For this review, take the finished solid that the model builds, in its own axes (mm). A direction names the side the tool comes from. Round coordinates to 2 decimals unless told otherwise and drop trailing zeros. Write each loop counter-clockwise with the first axis right and the second up, starting at its lowest first coordinate (ties: lowest second). Pieces come first, ordered by that corner, then holes. Notation, with made-up numbers: M 37.25,19 L 69.25,19 A14 cw 69.25,24 Z; hole C 42.5,-8 d6. An arc over 180 degrees is marked long. Write each question's results on one line, items separated by ' | '. Start each with the question number.
```python
from build123d import *

# Parameters (mm, degrees)
SKETCH1_R                = 6
SKETCH1_R_2              = 4.5
BOSS_EXTRUDE1_DEPTH      = 2
SKETCH1_5_R              = 21
SKETCH1_5_R_2            = 6
BOSS_EXTRUDE3_DEPTH      = 2.75
SKETCH2_R                = 1.75
CUT_EXTRUDE1_DEPTH       = 4.5
CIRPATTERN1_COUNT        = 3
SKETCH9_W                = 60
SKETCH9_H                = 11
BOSS_EXTRUDE7_DEPTH      = 15
BOSS_EXTRUDE7_DEPTH_BACK = 2.75
CUT_EXTRUDE3_REACH       = 13
SKETCH10_R               = 2.5
FILLET4_R                = 3
FILLET5_R                = 5


with BuildPart() as part:
    # Sketch1 → Boss-Extrude1 (new body)
    with BuildSketch(Plane(origin=(0, 0, 0), x_dir=(1, 0, 0), z_dir=(0, 1, 0))):
        Circle(SKETCH1_R)
        Circle(SKETCH1_R_2, mode=Mode.SUBTRACT)
    extrude(amount=BOSS_EXTRUDE1_DEPTH)

    # Sketch1<5> → Boss-Extrude3 (add)
    with BuildSketch(Plane(origin=(0, 0, 0), x_dir=(1, 0, 0), z_dir=(0, 1, 0))):
        Circle(SKETCH1_5_R)
        Circle(SKETCH1_5_R_2, mode=Mode.SUBTRACT)
    extrude(amount=BOSS_EXTRUDE3_DEPTH)

    # Sketch2 → Cut-Extrude1 (cut)
    with BuildSketch(Plane(origin=(0, 2.75, 0), x_dir=(1, 0, 0), z_dir=(0, 1, 0))):
        with Locations((0, -13.5)):
            Circle(SKETCH2_R)
    cut_extrude1 = extrude(amount=-CUT_EXTRUDE1_DEPTH, mode=Mode.SUBTRACT)

    # CirPattern1: Cut-Extrude1 ×3 about axis
    cirpattern1_axis = Axis((0, 0, 0), (0, 1, 0))
    for i in range(1, CIRPATTERN1_COUNT):
        add(cut_extrude1.rotate(cirpattern1_axis, i * 360 / CIRPATTERN1_COUNT), mode=Mode.SUBTRACT)

    # Sketch9 → Boss-Extrude7 (add, two sides)
    with BuildSketch(Plane.XZ) as boss_extrude7_sk:
        with Locations((0, -19.5)):
            Rectangle(SKETCH9_W, SKETCH9_H)
    extrude(amount=BOSS_EXTRUDE7_DEPTH)
    extrude(boss_extrude7_sk.sketch, amount=-BOSS_EXTRUDE7_DEPTH_BACK)

    # Sketch10 → Cut-Extrude3 (cut, up to next)
    with BuildSketch(Plane.XY.offset(-14), mode=Mode.PRIVATE) as cut_extrude3_sk1:
        with Locations((-18, -7.5)):
            Circle(SKETCH10_R)
    cut_extrude3_tool1 = extrude(cut_extrude3_sk1.sketch, amount=-CUT_EXTRUDE3_REACH, mode=Mode.PRIVATE) & part.part
    add(cut_extrude3_tool1.solids().sort_by_distance((-18, -7.5, -14))[0], mode=Mode.SUBTRACT)
    # Sketch10 → Cut-Extrude3 (cut, up to next)
    with BuildSketch(Plane.XY.offset(-14), mode=Mode.PRIVATE) as cut_extrude3_sk2:
        with Locations((18, -7.5)):
            Circle(SKETCH10_R)
    cut_extrude3_tool2 = extrude(cut_extrude3_sk2.sketch, amount=-CUT_EXTRUDE3_REACH, mode=Mode.PRIVATE) & part.part
    add(cut_extrude3_tool2.solids().sort_by_distance((18, -7.5, -14))[0], mode=Mode.SUBTRACT)

    # Fillet4
    fillet4_edges = [part.edges().sort_by_distance(p)[0] for p in [
        (-30, -6.125, -14),
        (30, -6.125, -14),
    ]]
    fillet(fillet4_edges, radius=FILLET4_R)

    # Fillet5
    fillet5_edges = [part.edges().sort_by_distance(p)[0] for p in [
        (-15.652475842, 1.375, -14),
        (15.652475842, 1.375, -14),
    ]]
    fillet(fillet5_edges, radius=FILLET5_R)


solid = part.part
```
Item 1: We need section D-D on x = 18. State the section outline as (y, z) points, then the cut area to 3 significant figures.
Item 2: We need section A-A on x = 0. State the section outline as (y, z) points.
Item 3: For probe 1 along Z at (x, y) = (0, 2.35); probe 2 along X at (y, z) = (-7.25, -21); probe 3 along Z at (x, y) = (0, 0.65), list the stretches that pass through material, from the lowest coordinate up.
Item 4: We need section B-B on z = 2.5. State the section outline as (x, y) points.
Item 5: Mouldability with a two-part tool opening along Y and no side actions: class faces 1 (the cylindrical face through (-29.14, -6, -14.9)), 2 (the cylindrical face through (15.5, -7.4, -19.4)), 3 (the flat face through (-1.4, 2, -4.5)) as pulls with the +Y half, pulls with the -Y half, needs draft (parallel to the pull), parting line crosses it, or undercut.
Item 6: Insertion check: P1, Ø5, axis at y = -10.5, z = -12, coming from the +X side; P2, Ø19, axis at x = 0, z = 0, coming from the -Y side; P3, Ø6, axis at x = 18, y = -7.5, coming from the +Z side; P4, Ø3, axis at x = -18, y = -7.5, coming from the +Z side. Each pin has a flat end and moves straight along its axis. Give the tip position at first contact, or say it passes through.
Item 7: We need section C-C on y = -7.5. State the section outline as (x, z) points.
Item 8: For faces 4 (the cylindrical face through (-5.994, 2.37, -0.264)), 5 (the flat face through (30, -6, -21)), list the 3-axis set-ups (+Z, -Z, +X, -X, +Y, -Y) from which the entire face can be reached by the end or side of a thin tool; tool diameter is ignored.
Numbers:
1) outline: M -15,-25 L -10,-25 L -10,-14 L -15,-14 Z; M -5,-25 L 2.75,-25 L 2.75,10.82 L 0,10.82 L 0,-14 L -5,-14 Z | area: 208 mm^2
2) outline: M -15,-25 L 2.75,-25 L 2.75,-6 L 2,-6 L 2,-4.5 L 0,-4.5 L 0,-14 L -15,-14 Z; M 0,4.5 L 2,4.5 L 2,6 L 2.75,6 L 2.75,11.75 L 0,11.75 Z; M 0,15.25 L 2.75,15.25 L 2.75,21 L 0,21 Z
3) probe 1: z = -25 to -6, 6 to 11.75, 15.25 to 21 | probe 2: x = -30 to -20.49, -15.51 to 15.51, 20.49 to 30 | probe 3: z = -25 to -4.5, 4.5 to 11.75, 15.25 to 21
4) outline: M -20.85,0 L -3.74,0 L -3.74,2 L -5.45,2 L -5.45,2.75 L -20.85,2.75 Z; M 3.74,0 L 20.85,0 L 20.85,2.75 L 5.45,2.75 L 5.45,2 L 3.74,2 Z
5) face 1: needs draft | face 2: undercut | face 3: pulls with the +Y half
6) P1: stops at x = 28.66 | P2: stops at y = 0 | P3: stops at z = -14 | P4: passes through
7) outline: M -30,-25 L -20.5,-25 L -20.5,-14 L -27,-14 A3 ccw -30,-17 Z; M -15.5,-25 L 15.5,-25 L 15.5,-14 L -15.5,-14 Z; M 20.5,-25 L 30,-25 L 30,-17 A3 ccw 27,-14 L 20.5,-14 Z
8) face 4: +Y | face 5: +Z, -Z, +X, +Y, -Y
